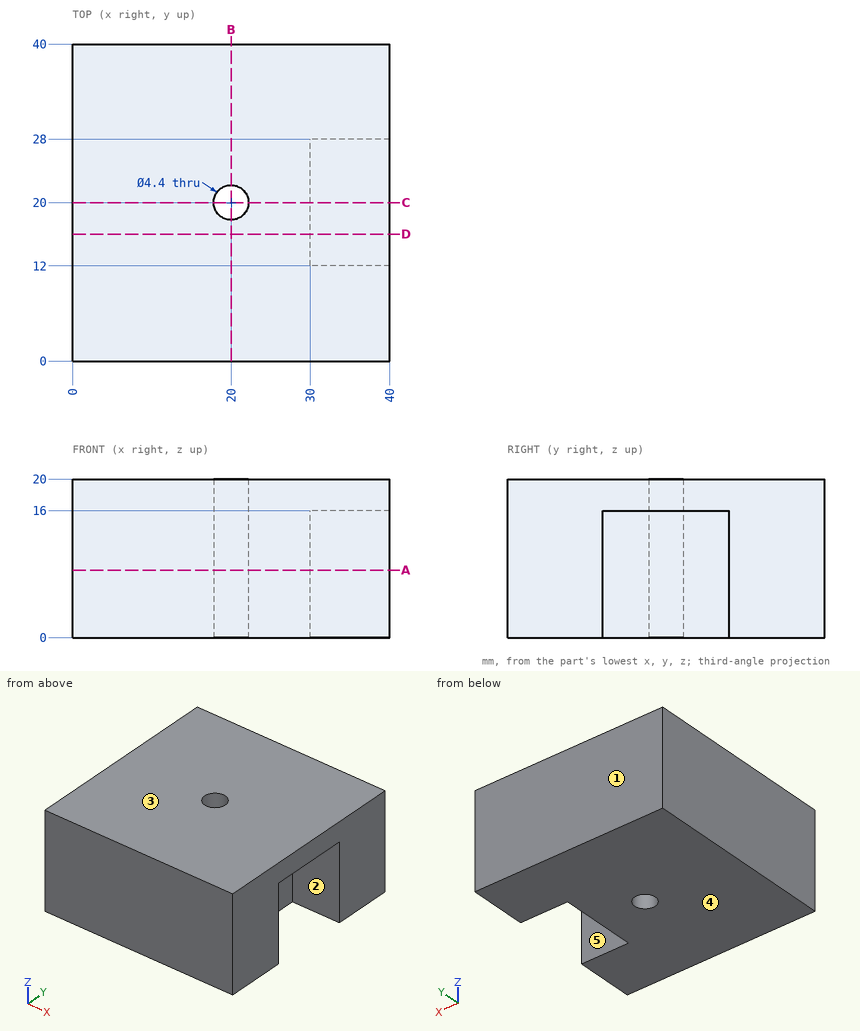
Answer from the drawing. Dimensions are ordinates in mm from the lowest x, y and z of the part. A direction names the side the tool comes from. Give positions to 0.01 mm unless a question says otherwise; leave off trailing zeros. Loops run counter-clockwise (first coordinate to the right, second up) from the corner with the lowest first, then second, coordinate; pieces in that order, holes last. Notation, with made-up numbers: (26.5, 24.25) - (33.5, 24.25) arc R20 ccw to (33.5, 42.25) - close; hole circle Ø9 at (85, 78.5). An arc over 180 degrees is marked (long way). Write each question's results on one line, items separated by ' | '.
1. Find section D-D, the plane y = 16. Write down the section's boundary in (x, z), then the cut area to 3 significant figures.
Resolved:
outline: (0, 0) - (30, 0) - (30, 16) - (40, 16) - (40, 20) - (0, 20) - close | area: 640 mm^2
2. Which of the six approach directions +Z, -Z, +X, -X, +Y, -Y give full straight-line access (tool end or side, diameter ignored) to the marked faces 4 and 5?
Resolved:
face 4: -Z, +X, -X, +Y, -Y | face 5: -Z, +X
3. Consider probe 1 along Y at (x, z) = (20, 15.5); probe 2 along Y at (x, z) = (38.5, 5); probe 3 along X at (y, z) = (26, 6.5). Determine where each line is inside the solid, lowest interval first. Write a range as from..to.
Resolved:
probe 1: y = 0..17.8, 22.2..40 | probe 2: y = 0..12, 28..40 | probe 3: x = 0..30
4. For a pull along Y with two mould halves and no side action, classify the marked faces 1, 2 and 3 as +Y half, -Y half, draft (parallel to the pull), parting line (faces both ways), or undercut.
Resolved:
face 1: +Y half | face 2: undercut | face 3: draft
5. Find section A-A, the plane z = 8.5. Write down the section's boundary in (x, y).
Resolved:
outline: (0, 0) - (40, 0) - (40, 12) - (30, 12) - (30, 28) - (40, 28) - (40, 40) - (0, 40) - close; hole circle Ø4.4 at (20, 20)
6. Flat-ended cylindrical pins translate along their axes: P1, Ø5, axis at x = 34.5, y = 17.5, coming from the -Z side; P2, Ø8, axis at y = 23.5, z = 5.5, coming from the +X side. Find the tip coordinate at first contact, or state that the pin passes through.
Resolved:
P1: stops at z = 16 | P2: stops at x = 30
7. Find section C-C, the plane y = 20. Write down the section's boundary in (x, z), then the cut area to 3 significant figures.
Resolved:
outline: (0, 0) - (17.8, 0) - (17.8, 20) - (0, 20) - close; (22.2, 0) - (30, 0) - (30, 16) - (40, 16) - (40, 20) - (22.2, 20) - close | area: 552 mm^2
8. Find section B-B, the plane x = 20. Write down the section's boundary in (y, z).
Resolved:
outline: (0, 0) - (17.8, 0) - (17.8, 20) - (0, 20) - close; (22.2, 0) - (40, 0) - (40, 20) - (22.2, 20) - close
